Geometry: final body of the model. Coordinates: model frame, mm. A direction names the side the tool comes from. Round coordinates to 2 decimals unless told otherwise and drop trailing zeros. Loops run counter-clockwise (first coordinate to the right, second up) from the corner with the lowest first, then second, coordinate; pieces in that order, holes last. Notation, with made-up numbers: M -8,3 L 4,3 A30 ccw 4,39 Z; hole C -29,20.5 d7. An arc over 180 degrees is marked long. Write each question's results on one line, items separated by ' | '.
```python
from build123d import *

# Parameters (mm, degrees)
F2_SIZE = 3
F3_SIZE = 1
F4_R    = 0.5


with BuildPart() as f1:
    # F0 (on Front) → F1 (revolve)
    with BuildSketch(Plane.XZ):
        Polygon((-7, 21), (0, 21), (0, 30), (7, 30), (7, 35), (23, 35), (23, 40), (0, 40), (0, 37), (-7, 37), align=None)
    revolve(axis=Axis((-3.5, 0, 0), (1, 0, 0)))

    # F2
    f2_edges = [f1.edges().sort_by_distance(p)[0] for p in [
        (-7, 0, -37),
    ]]
    chamfer(f2_edges, length=F2_SIZE)

    # F3
    f3_edges = [f1.edges().sort_by_distance(p)[0] for p in [
        (23, 0, -40),
        (23, 0, -35),
        (7, 0, -30),
    ]]
    chamfer(f3_edges, length=F3_SIZE)

    # F4
    f4_edges = [f1.edges().sort_by_distance(p)[0] for p in [
        (0, 0, -30),
        (7, 0, -35),
    ]]
    fillet(f4_edges, radius=F4_R)


solid = f1.part
```
1. Pin query (flat end, axial travel): P1, Ø12, axis at x = 8.5, z = -17.5, coming from the -Y side; P2, Ø1.5, axis at x = 13, z = 23, coming from the +Y side; P3, Ø3, axis at x = 18, z = -16, coming from the -Y side. Return the tip coordinate at first contact, or that it passes through.
Answer key:
P1: stops at y = -38.31 | P2: stops at y = 33.24 | P3: stops at y = -37.28
2. Access query for faces 5 (the face through (-2.03, 36.12, -8.02)), 6 (the face through (10.85, 39.05, -8.67)), 7 (the face through (7, -18, 26)). Directions: +Z, -Z, +X, -X, +Y, -Y. A direction counts if a zero-diameter tool reaches every point of the face in a straight line with its end or side. Return the directions, or none.
Answer key:
face 5: -X | face 6: +X, -X | face 7: +X
3. Section C-C (x = 2.5). Output: boundary loops of the cut face in (y, z), then the cut area to 3 significant figures.
Answer key:
outline: C 0,0 d80; hole C 0,0 d60 | area: 2,200 mm²
4. Draft query along Z for faces 1 (the face through (-7, -16, 15)), 2 (the face through (-6.85, 20.78, -27.1)), 3 (the face through (0, -20, 7)), 4 (the face through (15, 21, -28)). Return one class per face: pulls with the +Z half, pulls with the -Z half, needs draft (parallel to the pull), parting line crosses it, or undercut.
Answer key:
face 1: needs draft | face 2: parting line crosses it | face 3: undercut | face 4: undercut
5. Ray query, probe 1 along Y at (x, z) = (4.6, 0); probe 2 along Z at (x, y) = (13.5, 0). Return the intervals inside material, ascending.
Answer key:
probe 1: y = -40 to -30, 30 to 40 | probe 2: z = -40 to -35, 35 to 40
6. Section D-D (x = -2). Output: boundary loops of the cut face in (y, z), then the cut area to 3 significant figures.
Answer key:
outline: C 0,0 d74; hole C 0,0 d42 | area: 2,920 mm²
